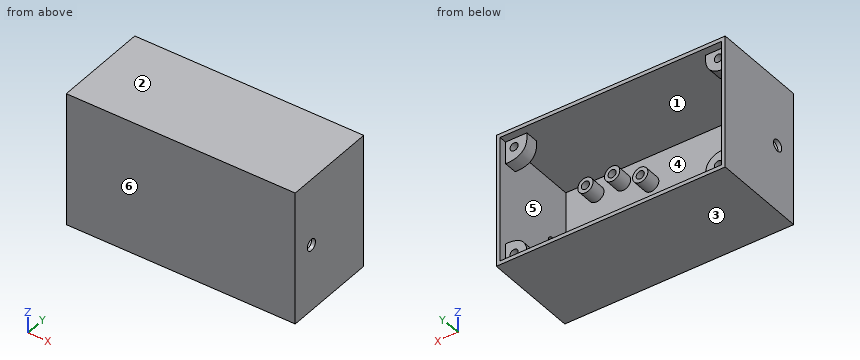
from build123d import *

# Parameters (mm, degrees)
SKETCH1_W           = 120
SKETCH1_H           = 70
BOSS_EXTRUDE1_DEPTH = 50
SKETCH4_W           = 116
SKETCH4_H           = 66
CUT_EXTRUDE1_DEPTH  = 48
SKETCH7_R           = 4
SKETCH7_R_2         = 2.125
BOSS_EXTRUDE3_DEPTH = 8
SKETCH9_R           = 3
CUT_EXTRUDE2_DEPTH  = 3
CUT_EXTRUDE3_START  = -3
SKETCH10_R          = 3
CUT_EXTRUDE3_DEPTH  = 3
BOSS_EXTRUDE4_DEPTH = 7
SKETCH13_R          = 2.125
CUT_EXTRUDE4_DEPTH  = 5


with BuildPart() as part:
    # Sketch1 → Boss-Extrude1 (new body)
    with BuildSketch(Plane(origin=(0, 0, 0), x_dir=(1, 0, 0), z_dir=(0, 1, 0))):
        Rectangle(SKETCH1_W, SKETCH1_H)
    extrude(amount=BOSS_EXTRUDE1_DEPTH)

    # Sketch4 → Cut-Extrude1 (cut)
    with BuildSketch(Plane(origin=(0, 50, 0), x_dir=(1, 0, 0), z_dir=(0, 1, 0))):
        Rectangle(SKETCH4_W, SKETCH4_H)
    extrude(amount=-CUT_EXTRUDE1_DEPTH, mode=Mode.SUBTRACT)

    # Sketch7 → Boss-Extrude3 (add)
    # profile 1 of 8: a face of its own
    with BuildSketch(Plane(origin=(0, 2, 0), x_dir=(1, 0, 0), z_dir=(0, 1, 0))):
        with Locations(Location((41.989163704, 23.984280939, 0), (0, 0, 270))):
            Circle(SKETCH7_R)
        with Locations(Location((41.989163704, 23.984280939, 0), (0, 0, 270))):
            Circle(SKETCH7_R_2, mode=Mode.SUBTRACT)
    # profile 2 of 8: a face of its own
    with BuildSketch(Plane(origin=(0, 2, 0), x_dir=(1, 0, 0), z_dir=(0, 1, 0))):
        with Locations(Location((27.989163704, 23.984280939, 0), (0, 0, 270))):
            Circle(SKETCH7_R)
        with Locations(Location((27.989163704, 23.984280939, 0), (0, 0, 270))):
            Circle(SKETCH7_R_2, mode=Mode.SUBTRACT)
    # profile 3 of 8: a face of its own
    with BuildSketch(Plane(origin=(0, 2, 0), x_dir=(1, 0, 0), z_dir=(0, 1, 0))):
        with Locations(Location((27.989163704, -25.015719061, 0), (0, 0, 270))):
            Circle(SKETCH7_R)
        with Locations(Location((27.989163704, -25.015719061, 0), (0, 0, 270))):
            Circle(SKETCH7_R_2, mode=Mode.SUBTRACT)
    # profile 4 of 8: a face of its own
    with BuildSketch(Plane(origin=(0, 2, 0), x_dir=(1, 0, 0), z_dir=(0, 1, 0))):
        with Locations(Location((41.989163704, -25.015719061, 0), (0, 0, 270))):
            Circle(SKETCH7_R)
        with Locations(Location((41.989163704, -25.015719061, 0), (0, 0, 270))):
            Circle(SKETCH7_R_2, mode=Mode.SUBTRACT)
    # profile 5 of 8: a face of its own
    with BuildSketch(Plane(origin=(0, 2, 0), x_dir=(1, 0, 0), z_dir=(0, 1, 0))):
        with Locations(Location((13.265207025, -17.861812849, 0), (0, 0, 270))):
            Circle(SKETCH7_R)
        with Locations(Location((13.265207025, -17.861812849, 0), (0, 0, 270))):
            Circle(SKETCH7_R_2, mode=Mode.SUBTRACT)
    # profile 6 of 8: a face of its own
    with BuildSketch(Plane(origin=(0, 2, 0), x_dir=(1, 0, 0), z_dir=(0, 1, 0))):
        with Locations(Location((13.265207025, 17.388187151, 0), (0, 0, 270))):
            Circle(SKETCH7_R)
        with Locations(Location((13.265207025, 17.388187151, 0), (0, 0, 270))):
            Circle(SKETCH7_R_2, mode=Mode.SUBTRACT)
    # profile 7 of 8: a face of its own
    with BuildSketch(Plane(origin=(0, 2, 0), x_dir=(1, 0, 0), z_dir=(0, 1, 0))):
        with Locations(Location((-46.734792975, 17.388187151, 0), (0, 0, 270))):
            Circle(SKETCH7_R)
        with Locations(Location((-46.734792975, 17.388187151, 0), (0, 0, 270))):
            Circle(SKETCH7_R_2, mode=Mode.SUBTRACT)
    # profile 8 of 8: a face of its own
    with BuildSketch(Plane(origin=(0, 2, 0), x_dir=(1, 0, 0), z_dir=(0, 1, 0))):
        with Locations(Location((-46.734792975, -17.861812849, 0), (0, 0, 270))):
            Circle(SKETCH7_R)
        with Locations(Location((-46.734792975, -17.861812849, 0), (0, 0, 270))):
            Circle(SKETCH7_R_2, mode=Mode.SUBTRACT)
    extrude(amount=BOSS_EXTRUDE3_DEPTH)

    # Sketch9 → Cut-Extrude2 (cut)
    with BuildSketch(Plane(origin=(60, 0, 0), x_dir=(0, 0, -1), z_dir=(1, 0, 0))):
        with Locations((0, 11.776029547)):
            Circle(SKETCH9_R)
    extrude(amount=-CUT_EXTRUDE2_DEPTH, mode=Mode.SUBTRACT)

    # Sketch10 → Cut-Extrude3 (cut)
    with BuildSketch(Plane.ZY.offset(60).offset(CUT_EXTRUDE3_START)):
        with Locations(Location((0, 11.776029547, 0), (0, 0, 180))):
            Circle(SKETCH10_R)
    extrude(amount=CUT_EXTRUDE3_DEPTH, mode=Mode.SUBTRACT)

    # Sketch12 → Boss-Extrude4 (add)
    with BuildSketch(Plane(origin=(0, 39, 0), x_dir=(1, 0, 0), z_dir=(0, 1, 0))):
        with BuildLine():
            Line((-46.836696193, -33), (-58, -33))
            Line((-58, -33), (-58, -21.439980772))
            add(Edge.make_bspline(
                [(-46.836696193, -33), (-45.747371945, -21.068063371), (-58, -21.439980772)],
                knots=[0, 0, 0, 1, 1, 1], degree=2))
        make_face()
        with BuildLine():
            Line((46.836696193, -33), (58, -33))
            Line((58, -33), (58, -21.439980772))
            add(Edge.make_bspline(
                [(46.836696193, -33), (45.747371945, -21.068063371), (58, -21.439980772)],
                knots=[0, 0, 0, 1, 1, 1], degree=2))
        make_face()
        with BuildLine():
            Line((58, 21.439980772), (58, 33))
            Line((58, 33), (46.836696193, 33))
            add(Edge.make_bspline(
                [(46.836696193, 33), (45.747371945, 21.068063371), (58, 21.439980772)],
                knots=[0, 0, 0, 1, 1, 1], degree=2))
        make_face()
        with BuildLine():
            Line((-46.836696193, 33), (-58, 33))
            Line((-58, 33), (-58, 21.439980772))
            add(Edge.make_bspline(
                [(-46.836696193, 33), (-45.747371945, 21.068063371), (-58, 21.439980772)],
                knots=[0, 0, 0, 1, 1, 1], degree=2))
        make_face()
    extrude(amount=BOSS_EXTRUDE4_DEPTH)

    # Sketch13 → Cut-Extrude4 (cut)
    with BuildSketch(Plane(origin=(0, 46, 0), x_dir=(1, 0, 0), z_dir=(0, 1, 0))):
        with Locations(Location((-53.5, -28.5, 0), (0, 0, 270))):
            Circle(SKETCH13_R)
        with Locations(Location((-53.5, 28.5, 0), (0, 0, 270))):
            Circle(SKETCH13_R)
        with Locations(Location((53.5, -28.5, 0), (0, 0, 270))):
            Circle(SKETCH13_R)
        with Locations(Location((53.5, 28.5, 0), (0, 0, 270))):
            Circle(SKETCH13_R)
    extrude(amount=-CUT_EXTRUDE4_DEPTH, mode=Mode.SUBTRACT)


solid = part.part
Verification items for the finished model (mm, model axes). Face numbers are marked on the shaded views. A direction names the side the tool comes from. Round coordinates to 2 decimals unless told otherwise and drop trailing zeros. Loops run counter-clockwise (first coordinate to the right, second up) from the corner with the lowest first, then second, coordinate; pieces in that order, holes last. Notation, with made-up numbers: (55.5, 49) - (97.5, 49) arc R22 ccw to (97.5, 58) - close; hole circle Ø11 at (58.5, 66). An arc over 180 degrees is marked (long way). Answer in a Markdown table with one row per item. Add a question column.
Q1. Section check D-D on z = -17. Enter the section's corners in (x, y).
Q2. Gauge pin test, flat ends, axial feed: pin 1 (5 mm diameter, centred on x = -53.5, z = 28.5, fed in from -Y); pin 2 (5 mm diameter, centred on x = -46.73, z = -17.39, fed in from +Y); pin 3 (5.5 mm diameter, centred on x = 50, z = 25, fed in from +Y); pin 4 (1.5 mm diameter, centred on x = -45.5, z = -2.5, fed in from +Y). Record the tip position at first contact, or that the pin passes through.
Q3. Material ranges on line 1 (X direction, y = 30, z = -1.5); line 2 (Z direction, x = -45.5, y = 18.5); line 3 (X direction, y = 43.25, z = -28.5) (3 decimals), recorded low to high.
Q4. Section check B-B on y = 17. Enter the section's corners in (x, z), plus the area to 3 significant figures.
Q5. Section check A-A on z = 0. Enter the section's corners in (x, y), plus the area to 3 significant figures.
Q6. Section check C-C on x = -15. Enter the section's corners in (y, z), plus the area to 3 significant figures.
Q7. Tool access check on the marked faces 1 and 2. Record the directions out of +Z, -Z, +X, -X, +Y, -Y that give a thin tool (end or side, any length) a straight path to the whole face; none if there is none.
Q8. Release check for a two-part mould opening along Z. For the marked faces 3, 4, 5 and 6 record: pulls with the +Z half, pulls with the -Z half, needs draft (parallel to the pull), parting line crosses it, or undercut.
Found:
| question | item | result |
|---|---|---|
| 1 | outline | (-60, 0) - (60, 0) - (60, 50) - (58, 50) - (58, 2) - (17.25, 2) - (17.25, 10) - (15.35, 10) - (15.35, 2) - (11.18, 2) - (11.18, 10) - (9.28, 10) - (9.28, 2) - (-42.75, 2) - (-42.75, 10) - (-44.65, 10) - (-44.65, 2) - (-48.82, 2) - (-48.82, 10) - (-50.72, 10) - (-50.72, 2) - (-58, 2) - (-58, 50) - (-60, 50) - close |
| 2 | pin 1 | stops at y = 0 |
| 2 | pin 2 | stops at y = 10 |
| 2 | pin 3 | stops at y = 46 |
| 2 | pin 4 | stops at y = 2 |
| 3 | line 1 | x = -60 to -58, 58 to 60 |
| 3 | line 2 | z = -35 to -33, 33 to 35 |
| 3 | line 3 | x = -60 to -55.625, -51.375 to -46.973, 46.973 to 51.375, 55.625 to 60 |
| 4 | outline | (-60, -35) - (60, -35) - (60, 35) - (-60, 35) - close; hole (-58, -33) - (58, -33) - (58, 33) - (-58, 33) - close |
| 4 | area | 744 mm² |
| 5 | outline | (-60, 0) - (60, 0) - (60, 8.78) - (58, 8.78) - (58, 2) - (-58, 2) - (-58, 8.78) - (-60, 8.78) - close; (-60, 14.78) - (-58, 14.78) - (-58, 50) - (-60, 50) - close; (58, 14.78) - (60, 14.78) - (60, 50) - (58, 50) - close |
| 5 | area | 408 mm² |
| 6 | outline | (0, -35) - (50, -35) - (50, -33) - (2, -33) - (2, 33) - (50, 33) - (50, 35) - (0, 35) - close |
| 6 | area | 332 mm² |
| 7 | face 1 | none |
| 7 | face 2 | +Z, +X, -X, +Y, -Y |
| 8 | face 3 | pulls with the -Z half |
| 8 | face 4 | undercut |
| 8 | face 5 | undercut |
| 8 | face 6 | needs draft |
